Read the model definition and answer for the solid it produces. Units are mm, in the model's axes. A direction names the side the tool comes from. Give positions to 0.01 mm unless a question says otherwise; leave off trailing zeros. Loops run counter-clockwise (first coordinate to the right, second up) from the corner with the lowest first, then second, coordinate; pieces in that order, holes last.
(1) Find section B-B, the plane z = 14. Write down the section's boundary in (x, y).
(2) Find section C-C, the plane y = -60.5. Write down the section's boundary in (x, z).
(3) This flat-tipped pin is pushed along its axis until it touches: P1, Ø8, axis at y = -91, z = 16, coming from the +X side. Where does it stop, or does it pass through?
(4) Which of the six approach directions +Z, -Z, +X, -X, +Y, -Y give full straight-line access (tool end or side, diameter ignored) to faces 1 (the face through (-58, 4, 19.05)), 2 (the face through (-57.15, -3, 9))?
(5) Find section A-A, the plane x = -27.5. Write down the section's boundary in (y, z).
(6) Straight lines are drawn through the part: probe 1 along Y at (x, z) = (28, 7.25); probe 2 along X at (y, z) = (95, 7). For each, find the intervals that lie inside material, in ascending order.
(7) Determine the mould class of faces 3 (the face through (2, 279.4, 9)), 4 (the face through (34, 209.55, 9)), 5 (the face through (127, 244, 9)), 6 (the face through (-2, -279.4, 9)) for opening direction Y: pulls with the +Y half, pulls with the -Y half, needs draft (parallel to the pull), parting line crosses it, or undercut.
```python
from build123d import *

# Parameters (mm, degrees)
F1_DEPTH = 19.05


with BuildPart() as f1:
    # F0 (on Top) → F1 (new body)
    with BuildSketch(Plane.XY):
        Polygon((-57.15, -209.55), (-127, -209.55), (-127, -279.4), (127, -279.4), (127, -209.55), align=None)
        Polygon((127, 279.4), (-127, 279.4), (-127, -209.55), (-57.15, -209.55), (-57.15, 209.55), (127, 209.55), align=None)
    extrude(amount=F1_DEPTH)


solid = f1.part
```
Entries:
1. outline: (-127, -279.4) - (127, -279.4) - (127, -209.55) - (-57.15, -209.55) - (-57.15, 209.55) - (127, 209.55) - (127, 279.4) - (-127, 279.4) - close
2. outline: (-127, 0) - (-57.15, 0) - (-57.15, 19.05) - (-127, 19.05) - close
3. P1: stops at x = -57.15
4. face 1: +Z, +X, -X, +Y, -Y
4. face 2: +Z, -Z, +X
5. outline: (-279.4, 0) - (-209.55, 0) - (-209.55, 19.05) - (-279.4, 19.05) - close; (209.55, 0) - (279.4, 0) - (279.4, 19.05) - (209.55, 19.05) - close
6. probe 1: y = -279.4 to -209.55, 209.55 to 279.4
6. probe 2: x = -127 to -57.15
7. face 3: pulls with the +Y half
7. face 4: undercut
7. face 5: needs draft
7. face 6: pulls with the -Y half
